Input: part model. Units: mm. Frame: model coordinates. Face numbers are marked on the shaded views. Coordinates: 2 decimals unless noted, no trailing zeros. Loops run counter-clockwise (first coordinate to the right, second up) from the corner with the lowest first, then second, coordinate; pieces in that order, holes last.
(1) Section D-D, the plane z = 7.75. Return loops of the section in (x, y) (3 decimals).
(2) Contact query for flat-ended pins moving along their axis: P1, Ø0.9, axis at y = 15.5, z = 5.5, coming from the -X side; P2, Ø12.5, axis at x = -16.5, y = 16, coming from the -Z side; P3, Ø2, axis at y = 6, z = -3, coming from the -X side; P4, Ø2, axis at y = 13.5, z = 6.5, coming from the -X side. Output: stop coordinate, or through.
(3) Section C-C, the plane y = 10.5. Give the number of separate pieces and of enclosed holes in the cut face, then the cut area to 3 significant figures.
(4) Mould query, pull axis Z, two halves, no side actions, for the marked faces 1, 2 and 3. Classes: released by +Z, released by -Z, zero draft, split by the parting line, or undercut.
(5) Section B-B, the plane x = 2.54. Return loops of the section in (y, z).
(6) Section A-A, the plane x = 7. Return loops of the section in (y, z) (3 decimals), then the cut area to 3 significant figures.
(7) Line query: L1, parallel to X at y = 17.5, z = 1; L2, parallel to X at y = -2.3, z = 1.25; L3, parallel to Z at x = -9, y = 12.25. Output: solid intervals per line, ascending.
```python
from build123d import *
from build123d.topology import SkipClean

# Parameters (mm, degrees)
BOSS_EXTRUDE1_DEPTH     = 2.5
BOSS_EXTRUDE1_2_DEPTH   = 2.5
BOSS_EXTRUDE2_DEPTH     = 6.35
BOSS_EXTRUDE3_DEPTH     = 6.35
SKETCH4_R               = 3.175
CUT_EXTRUDE1_DEPTH      = 25.4
SKETCH5_R               = 1.5875
CUT_EXTRUDE2_DEPTH      = 25.4
CUT_EXTRUDE3_DEPTH      = 25.4
CUT_EXTRUDE4_REACH      = 43
CUT_EXTRUDE4_END_RADIUS = 3.175
CUT_EXTRUDE5_REACH      = 39.36
SKETCH8_W               = 2.54
SKETCH8_H               = 9.525
SKETCH9_W               = 0.7112
SKETCH9_H               = 15.2
BOSS_EXTRUDE4_DEPTH     = 17
BOSS_EXTRUDE5_DEPTH     = 1.016
SKETCH11_W              = 1.176658287
SKETCH11_H              = 2.5
SKETCH11_W_2            = 2.636987944
SKETCH11_H_2            = 15.2
BOSS_EXTRUDE6_DEPTH     = 1.27
CUT_EXTRUDE6_DEPTH      = 38.864332241
BOSS_EXTRUDE7_START     = 2.54
BOSS_EXTRUDE7_DEPTH     = 2.54
BOSS_EXTRUDE8_DEPTH     = 2.54
BOSS_EXTRUDE9_DEPTH     = 0.508
BOSS_EXTRUDE10_DEPTH    = 0.508
CUT_EXTRUDE7_DEPTH      = 3.81
CUT_EXTRUDE8_DEPTH      = 3.81
BOSS_EXTRUDE11_DEPTH    = 3.81


with BuildPart() as part:
    # Sketch1 → Boss-Extrude1 (new body)
    with BuildSketch(Plane.XY):
        Polygon((5.08, 0), (0, 0), (0, 19.141079028), (-1.033059908, 19.141079028), (-3.75575709, 23.125698967), (-8.376397661, 9.077684872), (-11.679025045, 6.820994294), (-21.26996, 20.857160675), (-22.86, 19.770683798), (-22.86, -3.81), (8.89, -3.81), (8.89, 24.384), (5.08, 24.384), align=None)
    extrude(amount=BOSS_EXTRUDE1_DEPTH)



with BuildPart() as body_2:
    # Sketch1 → Boss-Extrude1 2 (new body)
    with BuildSketch(Plane.XY):
        Polygon((-10.069369191, 23.749), (-4.328956497, 23.964566322), (-4.615556201, 24.384), (-16.108492032, 24.384), (-17.03780348, 23.749), align=None)
    extrude(amount=BOSS_EXTRUDE1_2_DEPTH)


with BuildPart() as part_1:
    add(part.part)

    add(body_2.part)  # Boss-Extrude2 merges body 2
    # Sketch2 → Boss-Extrude2 (add)
    with BuildSketch(Plane.XY.offset(2.5)):
        Polygon((-11.679025045, 6.820994294), (-21.26996, 20.857160675), (-22.86, 19.770683798), (-22.86, -3.81), (8.89, -3.81), (8.89, 24.384), (5.08, 24.384), (5.08, 0), (0, 0), (0, 19.141079028), (-1.033059908, 19.141079028), (-3.75575709, 23.125698967), (-8.376397661, 9.077684872), align=None)
        Polygon((-16.108492032, 24.384), (-18.00931945, 23.085161582), (-8.418384495, 9.048995201), (-8.376397661, 9.077684872), (-3.75575709, 23.125698967), (-1.033059908, 19.141079028), (0, 19.141079028), (0, 0), (5.08, 0), (5.08, 24.384), align=None)
    extrude(amount=BOSS_EXTRUDE2_DEPTH)

    # Sketch3 → Boss-Extrude3 (add)
    with BuildSketch(Plane(origin=(0, 0, 0), x_dir=(-1, 0, 0), z_dir=(0, 0, -1))):
        Polygon((-8.89, 24.384), (-8.89, -3.81), (22.86, -3.81), (22.86, 19.770683798), (21.26996, 20.857160675), (11.679025045, 6.820994294), (8.376397661, 9.077684872), (18.00931945, 23.085161582), (16.108492032, 24.384), align=None)
    extrude(amount=BOSS_EXTRUDE3_DEPTH)

    # Sketch4 → Cut-Extrude1 (cut)
    with BuildSketch(Plane(origin=(0, 24.384, 0), x_dir=(1, 0, 0), z_dir=(0, 1, 0))):
        with Locations(Location((2.54, -1.25, 0), (0, 0, 270))):
            Circle(SKETCH4_R)
    extrude(amount=-CUT_EXTRUDE1_DEPTH, mode=Mode.SUBTRACT)

    # Sketch5 → Cut-Extrude2 (cut)
    with BuildSketch(Plane(origin=(0, -1.016, 0), x_dir=(1, 0, 0), z_dir=(0, 1, 0))):
        with Locations(Location((2.54, -1.25, 0), (0, 0, 270))):
            Circle(SKETCH5_R)
    extrude(amount=-CUT_EXTRUDE2_DEPTH, mode=Mode.SUBTRACT)

    # Sketch6 → Cut-Extrude3 (cut)
    with BuildSketch(Plane.XY.offset(8.85)):
        Polygon((-22.86, 16.430904611), (-9.029357481, -3.81), (-22.86, -3.81), align=None)
    extrude(amount=-CUT_EXTRUDE3_DEPTH, mode=Mode.SUBTRACT)

    # Cut-Extrude4: up to this cylinder (the profile starts outside it)
    with SkipClean():  # the faces are left unmerged after this step: merging them gives an invalid solid
        cut_extrude4_end = Plane(origin=(2.54, 2.159, 1.25), z_dir=(0, 1, 0)) * Cylinder(CUT_EXTRUDE4_END_RADIUS, 96.045024, mode=Mode.PRIVATE)
        # Sketch7 → Cut-Extrude4 (cut, up to the surface)
        with BuildSketch(Plane(origin=(8.89, 0, 0), x_dir=(0, 0, -1), z_dir=(1, 0, 0)), mode=Mode.PRIVATE) as cut_extrude4_sk1:
            with BuildLine():
                ThreePointArc((1.925, 2.159), (-1.25, 5.334), (-4.425, 2.159))
                Line((-4.425, 2.159), (1.925, 2.159))
            make_face()
        cut_extrude4_tool1 = extrude(cut_extrude4_sk1.sketch, amount=-CUT_EXTRUDE4_REACH, mode=Mode.PRIVATE) - cut_extrude4_end
        add(cut_extrude4_tool1.solids().sort_by_distance((8.89, 3.506512, 1.25))[0], mode=Mode.SUBTRACT)
        # Sketch7 → Cut-Extrude4 (cut, up to the surface)
        with BuildSketch(Plane(origin=(8.89, 0, 0), x_dir=(0, 0, -1), z_dir=(1, 0, 0)), mode=Mode.PRIVATE) as cut_extrude4_sk2:
            with BuildLine():
                Line((1.925, 2.159), (-4.425, 2.159))
                ThreePointArc((-4.425, 2.159), (-3.49506403, -0.08606403), (-1.25, -1.016))
                ThreePointArc((-1.25, -1.016), (0.99506403, -0.08606403), (1.925, 2.159))
            make_face()
        cut_extrude4_tool2 = extrude(cut_extrude4_sk2.sketch, amount=-CUT_EXTRUDE4_REACH, mode=Mode.PRIVATE) - cut_extrude4_end
        add(cut_extrude4_tool2.solids().sort_by_distance((8.89, 0.811488, 1.25))[0], mode=Mode.SUBTRACT)
        # Sketch7 → Cut-Extrude4 (cut, up to the surface)
        with BuildSketch(Plane(origin=(8.89, 0, 0), x_dir=(0, 0, -1), z_dir=(1, 0, 0)), mode=Mode.PRIVATE) as cut_extrude4_sk3:
            with BuildLine():
                ThreePointArc((1.925, 2.159), (-1.25, 5.334), (-4.425, 2.159))
                Line((-4.425, 2.159), (1.925, 2.159))
            make_face()
        cut_extrude4_tool3 = extrude(cut_extrude4_sk3.sketch, amount=-CUT_EXTRUDE4_REACH, mode=Mode.PRIVATE) - cut_extrude4_end
        add(cut_extrude4_tool3.solids().sort_by_distance((8.89, 3.506512, 1.25))[0], mode=Mode.SUBTRACT)
        # Sketch7 → Cut-Extrude4 (cut, up to the surface)
        with BuildSketch(Plane(origin=(8.89, 0, 0), x_dir=(0, 0, -1), z_dir=(1, 0, 0)), mode=Mode.PRIVATE) as cut_extrude4_sk4:
            with BuildLine():
                Line((1.925, 2.159), (-4.425, 2.159))
                ThreePointArc((-4.425, 2.159), (-3.49506403, -0.08606403), (-1.25, -1.016))
                ThreePointArc((-1.25, -1.016), (0.99506403, -0.08606403), (1.925, 2.159))
            make_face()
        cut_extrude4_tool4 = extrude(cut_extrude4_sk4.sketch, amount=-CUT_EXTRUDE4_REACH, mode=Mode.PRIVATE) - cut_extrude4_end
        add(cut_extrude4_tool4.solids().sort_by_distance((8.89, 0.811488, 1.25))[0], mode=Mode.SUBTRACT)

    # Cut-Extrude5: up to this face of the body (flat: up to its plane)
    cut_extrude5_end = Plane(part_1.part.faces().sort_by_distance((4.72156403, -1.016, 3.43156403))[0])
    # Sketch8 → Cut-Extrude5 (cut, up to the picked face)
    with BuildSketch(Plane(origin=(0, 24.384, 0), x_dir=(1, 0, 0), z_dir=(0, 1, 0)), mode=Mode.PRIVATE) as cut_extrude5_sk1:
        with Locations((2.54, -1.25)):
            Rectangle(SKETCH8_W, SKETCH8_H)
    cut_extrude5_tool1 = split(extrude(cut_extrude5_sk1.sketch, amount=-CUT_EXTRUDE5_REACH, mode=Mode.PRIVATE), bisect_by=cut_extrude5_end, keep=Keep.BOTH, mode=Mode.PRIVATE)
    add(cut_extrude5_tool1.solids().sort_by(Axis((2.54, 24.384, 1.25), (0, -1, 0)))[0], mode=Mode.SUBTRACT)

    # Sketch9 → Boss-Extrude4 (add)
    with BuildSketch(Plane(origin=(-6.894633763, 10.090176515, 0), x_dir=(0.825656845959394, 0.5641726444275594, 0), z_dir=(-0.5641726444275594, 0.825656845959394, 0))):
        with Locations((-5.439048594, -1.25)):
            Rectangle(SKETCH9_W, SKETCH9_H)
        Polygon((-1.794648594, 6.35), (-2.302648594, 6.35), (-2.302648594, 1.6202), (-3.623501238, 1.6202), (-3.623501238, 0.7312), (-1.794648594, 0.7312), align=None)
        Polygon((-1.845501238, -8.85), (-1.845501238, -4.6028), (-3.572648594, -4.6028), (-3.572648594, -5.6188), (-2.683648594, -5.6188), (-2.683648594, -8.85), align=None)
    extrude(amount=BOSS_EXTRUDE4_DEPTH)

    # Sketch10 → Boss-Extrude5 (add)
    with BuildSketch(Plane(origin=(-6.894633763, 10.090176515, 0), x_dir=(0.8256568459593948, 0.5641726444275585, 0), z_dir=(-0.5641726444275585, 0.8256568459593948, 0))):
        Polygon((-5.083448594, -8.85), (-2.683648594, -8.85), (-2.683648594, -5.6188), (-3.572648594, -5.6188), (-3.572648594, -4.6028), (-1.845501238, -4.6028), (-1.845501238, -2.5), (-1.794648594, -2.5), (-1.794648594, 0), (-1.794648594, 0.7312), (-3.623501238, 0.7312), (-3.623501238, 1.6202), (-2.302648594, 1.6202), (-2.302648594, 6.35), (-5.083448594, 6.35), align=None)
    extrude(amount=BOSS_EXTRUDE5_DEPTH)

    # Sketch11 → Boss-Extrude6 (add)
    with BuildSketch(Plane(origin=(-16.485568719, 24.126342896, 0), x_dir=(0.8256568459593935, 0.5641726444275603, 0), z_dir=(-0.5641726444275603, 0.8256568459593935, 0))):
        with Locations((-1.257172095, -1.25)):
            Rectangle(SKETCH11_W, SKETCH11_H)
        Polygon((-3.623501238, 1.6202), (-3.623501238, 0.7312), (-1.845501238, 0.7312), (-1.845501238, 0), (-0.668842951, 0), (-0.668842951, -2.5), (-1.845501238, -2.5), (-1.845501238, -4.6028), (-3.572648594, -4.6028), (-3.572648594, -5.6188), (-2.683648594, -5.6188), (-2.683648594, -8.85), (0.456699038, -8.85), (0.456699038, 6.35), (-2.302648594, 6.35), (-2.302648594, 1.6202), align=None)
        with Locations((-6.401942566, -1.25)):
            Rectangle(SKETCH11_W_2, SKETCH11_H_2)
    extrude(amount=BOSS_EXTRUDE6_DEPTH)

    # Sketch12 → Cut-Extrude6 (cut, through all)
    with BuildSketch(Plane.XY.offset(8.85)):
        Polygon((-16.108492032, 24.384), (-18.359576008, 24.384), (-16.82499129, 25.432584194), align=None)
        Polygon((-22.86, 19.770683798), (-22.86, 21.308853083), (-23.576499258, 20.819267993), align=None)
    extrude(amount=-CUT_EXTRUDE6_DEPTH, mode=Mode.SUBTRACT)

    # Sketch13 → Boss-Extrude7 (add)
    with BuildSketch(Plane(origin=(0, 19.141079028, 0), x_dir=(1, 0, 0), z_dir=(0, 1, 0)).offset(BOSS_EXTRUDE7_START)):
        with BuildLine():
            Line((-0.378582704, 0), (-1.033059908, 0))
            Line((-1.033059908, 0), (-1.033059908, -2.5))
            Line((-1.033059908, -2.5), (-0.378582704, -2.5))
            ThreePointArc((-0.378582704, -2.5), (-0.635, -1.25), (-0.378582704, 0))
        make_face()
    extrude(amount=-BOSS_EXTRUDE7_DEPTH)

    # Sketch15 → Boss-Extrude8 (add)
    with BuildSketch(Plane.XY):
        Polygon((-4.156996675, 23.712906116), (-4.328956497, 23.964566322), (-4.808856613, 23.946544917), (-4.492543617, 23.483626353), align=None)
        Polygon((-3.75575709, 23.125698967), (-3.927716912, 23.377359173), (-4.263263855, 23.148079411), (-3.915700647, 22.639426706), align=None)
    extrude(amount=BOSS_EXTRUDE8_DEPTH)

    # Sketch16 → Boss-Extrude9 (add)
    with BuildSketch(Plane.XY):
        Polygon((-4.263263855, 23.148079411), (-4.492543617, 23.483626353), (-4.156996675, 23.712906116), (-3.927716912, 23.377359173), align=None)
    extrude(amount=BOSS_EXTRUDE9_DEPTH)

    # Sketch17 → Boss-Extrude10 (add)
    with BuildSketch(Plane(origin=(0, 0, 2.5), x_dir=(-1, 0, 0), z_dir=(0, 0, -1))):
        Polygon((4.263263855, 23.148079411), (4.492543617, 23.483626353), (4.156996675, 23.712906116), (3.927716912, 23.377359173), align=None)
    extrude(amount=BOSS_EXTRUDE10_DEPTH)

    # Sketch18 → Cut-Extrude7 (cut)
    with BuildSketch(Plane(origin=(0, 0, 2.5), x_dir=(-1, 0, 0), z_dir=(0, 0, -1))):
        Polygon((1.033059908, 24.384), (1.033059908, 21.681079028), (1.033059908, 19.141079028), (4.615556201, 24.384), align=None)
    extrude(amount=-CUT_EXTRUDE7_DEPTH, mode=Mode.SUBTRACT)

    # Sketch19 → Cut-Extrude8 (cut)
    with BuildSketch(Plane.XY):
        Polygon((-1.033059908, 19.141079028), (-1.033059908, 21.681079028), (-1.033059908, 24.384), (-4.615556201, 24.384), align=None)
    extrude(amount=-CUT_EXTRUDE8_DEPTH, mode=Mode.SUBTRACT)

    # Sketch20 → Boss-Extrude11 (add)
    with BuildSketch(Plane.XY):
        Polygon((-10.069369191, 23.749), (-4.492543617, 23.483626353), (-4.808856613, 23.946544917), align=None)
    extrude(amount=BOSS_EXTRUDE11_DEPTH)


solid = part_1.part
```
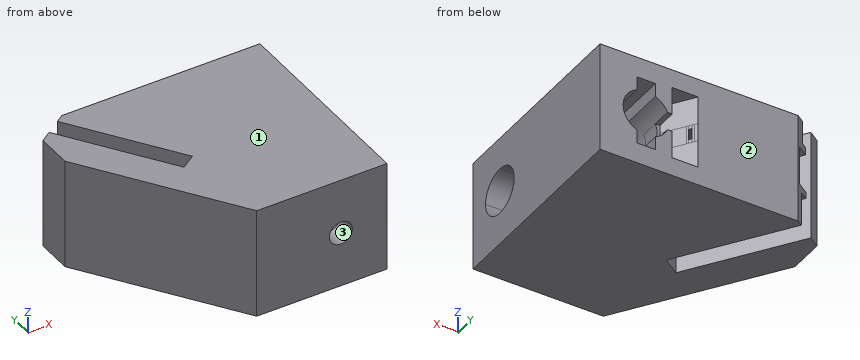
Report:
1. outline: (-22.86, 16.431) - (-9.029, -3.81) - (8.89, -3.81) - (8.89, 24.384) - (-18.36, 24.384) - (-19.418, 23.661) - (-9.684, 9.415) - (-11.665, 8.061) - (-21.399, 22.307) - (-22.86, 21.309) - close
2. P1: stops at x = -22.53
2. P2: stops at z = -6.35
2. P3: stops at x = -16.42
2. P4: stops at x = -21.54
3. separate pieces: 2
3. enclosed holes: 1
3. area: 327 mm2
4. face 1: released by +Z
4. face 2: zero draft
4. face 3: undercut
5. outline: (-3.81, -6.35) - (24.38, -6.35) - (24.38, -3.51) - (-1.02, -3.51) - (-1.02, -0.34) - (-3.81, -0.34) - close; (-3.81, 2.84) - (-1.02, 2.84) - (-1.02, 6.01) - (24.38, 6.01) - (24.38, 8.85) - (-3.81, 8.85) - close
6. outline: (-3.81, -6.35) - (24.384, -6.35) - (24.384, 8.85) - (-3.81, 8.85) - close; hole circle Ø6.35 at (2.159, 1.25)
6. area: 397 mm2
7. L1: x = -22.86 to -18.11, -5.61 to -0.63, 5.71 to 8.89
7. L2: x = -10.06 to 0.95, 4.13 to 8.89
7. L3: z = -6.35 to 0, 2.5 to 8.85
